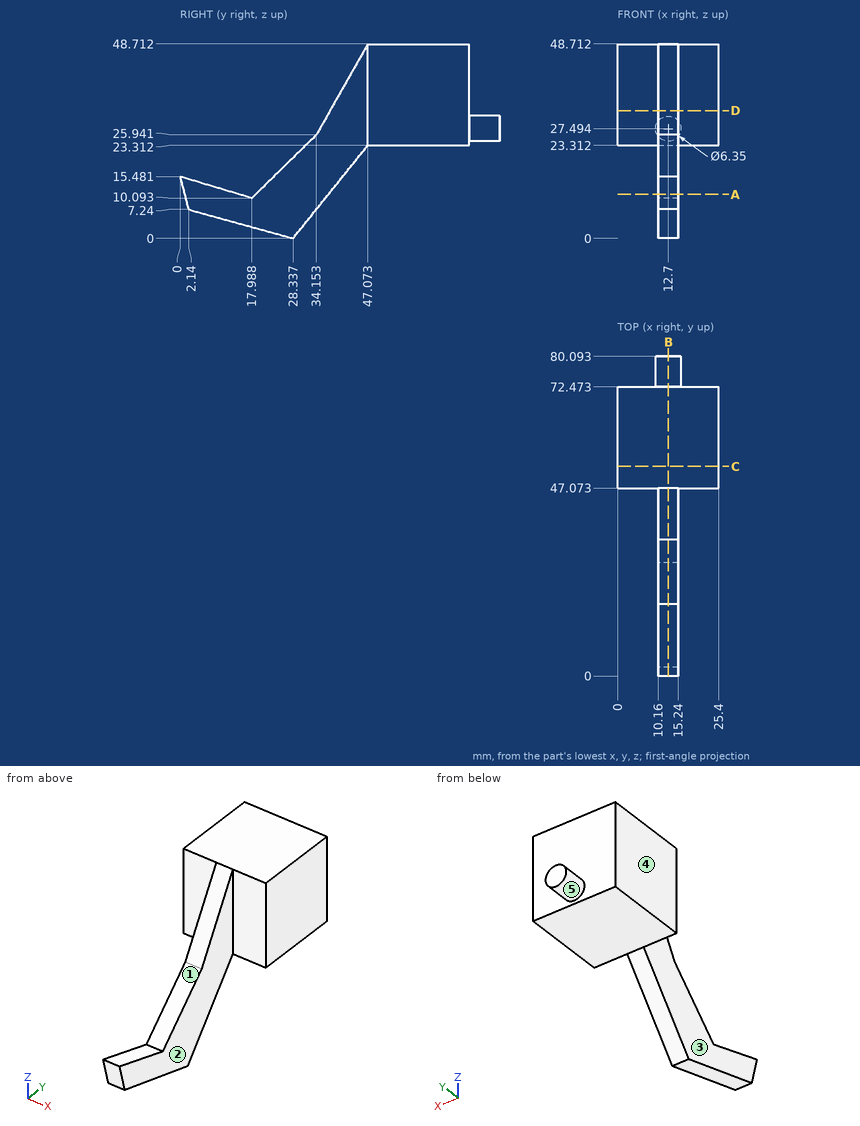
Design review of the part shown in the three views and the two pictorial views. Dimensions are in mm from the part's minimum x, y and z. A direction names the side the tool comes from. Give positions to 0.01 mm unless a question says otherwise; leave off trailing zeros. Write each loop counter-clockwise with the first axis right and the second up, starting at its lowest first coordinate (ties: lowest second). Pieces come first, ordered by that corner, then holes.
(1) Tool access review of the marked faces 1, 2, 3, 4 and 5: name each direction out of +Z, -Z, +X, -X, +Y, -Y from which nothing blocks a thin tool from reaching the whole face with its end or side.
Checked values:
face 1: +Z, +X, -X
face 2: +Z, -Z, +X, -Y
face 3: +Z, -Z, -X, -Y
face 4: +Z, -Z, -X, +Y, -Y
face 5: +Y
(2) Add section D-D (z = 32). Give the boundary of the cut face in (x, y).
Checked values:
outline: (0, 47.07) - (10.16, 47.07) - (10.16, 37.59) - (15.24, 37.59) - (15.24, 47.07) - (25.4, 47.07) - (25.4, 72.47) - (0, 72.47) - close
(3) Add section C-C (y = 52.5). Give the boundary of the cut face in (x, z), and give its area (3 significant figures).
Checked values:
outline: (0, 23.31) - (25.4, 23.31) - (25.4, 48.71) - (0, 48.71) - close
area: 645 mm2
(4) Clearance check with flat-ended pins moving along their axes: pin 1 Ø5 at (x, z) = (2.5, 41.5) entering from -Y; pin 2 Ø1.5 at (x, y) = (15, 57.5) entering from -Z; pin 3 Ø14 at (y, z) = (13.5, 13.5) entering from +X; pin 4 Ø12 at (y, z) = (58, 14.5) entering from +X. State where each tip first meets the part, or that it passes through.
Checked values:
pin 1: stops at y = 47.07
pin 2: stops at z = 23.31
pin 3: stops at x = 15.24
pin 4: passes through
(5) Add section A-A (z = 11). Give the boundary of the cut face in (x, y), and give its area (3 significant figures).
Checked values:
outline: (10.16, 1.16) - (15.24, 1.16) - (15.24, 14.96) - (10.16, 14.96) - close; (10.16, 18.91) - (15.24, 18.91) - (15.24, 37.18) - (10.16, 37.18) - close
area: 163 mm2
(6) Add section B-B (x = 12.7). Give the boundary of the cut face in (y, z), and give its area (3 significant figures).
Checked values:
outline: (0, 15.48) - (2.14, 7.24) - (28.34, 0) - (47.07, 23.31) - (72.47, 23.31) - (72.47, 24.32) - (80.09, 24.32) - (80.09, 30.67) - (72.47, 30.67) - (72.47, 48.71) - (47.07, 48.71) - (34.15, 25.94) - (17.99, 10.09) - close
area: 1,360 mm2
(7) Wall thickness on line 1 along Z through (x, y) = (5, 61.5); line 2 along X through (y, z) = (31, 15); line 3 along Y through (x, z) = (2.75, 29): over which ranges is each line inside the solid? List them lowest first.
Checked values:
line 1: z = 23.31 to 48.71
line 2: x = 10.16 to 15.24
line 3: y = 47.07 to 72.47
